Build history of the part. All positions in model axes, mm. A direction names the side the tool comes from. Round coordinates to 2 decimals unless told otherwise and drop trailing zeros. Write each loop counter-clockwise with the first axis right and the second up, starting at its lowest first coordinate (ties: lowest second). Pieces come first, ordered by that corner, then holes.
1) Saw through at D-D (z = 3.7). Write the cut outline in (x, y), plus the area to 3 significant figures.
2) Which spindle directions (+Z, -Z, +X, -X, +Y, -Y) get a long thin tool onto all of the face, cutting with end or side? Do faces 4 (the flat face through (12.3, -12.3, 3)), 5 (the cylindrical face through (-12.5, 11.07, 1.52)). Say none if no direction does.
3) Saw through at B-B (x = 0). Write the cut outline in (y, z), plus the area to 3 significant figures.
4) Flat gauge pins, fed straight in: pin 1 (2.5 mm diameter, centred on x = -11, y = -11, fed in from -Z); pin 2 (1.8 mm diameter, centred on x = 9.5, y = 10, fed in from +Z); pin 3 (8 mm diameter, centred on x = -11, y = 11, fed in from +Z). Where does each tip first touch, or does it go through?
5) Pull direction Y, two halves, no side cores. Call faces 1 (the flat face through (0, -15, 3)), 2 (the flat face through (-9.7, 9.7, 3)), 3 (the flat face through (0, 15, 3)): +Y half, -Y half, draft (parallel to the pull), parting line (faces both ways), or undercut.
6) Saw through at A-A (y = -11). Write the cut outline in (x, z).
7) Wall check: probe 1 along Y at (x, z) = (11, 5.25); probe 2 along Y at (x, z) = (-11, 1.45); probe 3 along X at (y, z) = (10.5, 1.65). Give the ranges that are in metal, low to high.
from build123d import *

# Parameters (mm, degrees)
SKETCH1_W           = 30
SKETCH1_H           = 30
SKETCH1_R           = 9.5
BOSS_EXTRUDE1_DEPTH = 6
SKETCH3_R           = 1.5
CUT_EXTRUDE2_DEPTH  = 7
SKETCH4_R           = 3
CUT_EXTRUDE3_DEPTH  = 3
FILLET1_R           = 3


with BuildPart() as part:
    # Sketch1 → Boss-Extrude1 (new body)
    with BuildSketch(Plane.XY):
        Rectangle(SKETCH1_W, SKETCH1_H)
        Circle(SKETCH1_R, mode=Mode.SUBTRACT)
    extrude(amount=BOSS_EXTRUDE1_DEPTH)

    # Sketch3 → Cut-Extrude2 (cut, through all)
    with BuildSketch(Plane.XY.offset(6)):
        with Locations((-11, 11)):
            Circle(SKETCH3_R)
        with Locations((11, 11)):
            Circle(SKETCH3_R)
        with Locations((11, -11)):
            Circle(SKETCH3_R)
        with Locations((-11, -11)):
            Circle(SKETCH3_R)
    extrude(amount=-CUT_EXTRUDE2_DEPTH, mode=Mode.SUBTRACT)

    # Sketch4 → Cut-Extrude3 (cut)
    with BuildSketch(Plane.XY.offset(6)):
        with Locations((-11, 11)):
            Circle(SKETCH4_R)
        with Locations((11, 11)):
            Circle(SKETCH4_R)
        with Locations((11, -11)):
            Circle(SKETCH4_R)
        with Locations((-11, -11)):
            Circle(SKETCH4_R)
    extrude(amount=-CUT_EXTRUDE3_DEPTH, mode=Mode.SUBTRACT)

    # Fillet1
    fillet1_edges = [part.edges().sort_by_distance(p)[0] for p in [
        (15, -15, 3),
        (-15, -15, 3),
        (-15, 15, 3),
        (15, 15, 3),
    ]]
    fillet(fillet1_edges, radius=FILLET1_R)


solid = part.part
Evaluation:
1. outline: (-15, -12) arc R3 ccw to (-12, -15) - (12, -15) arc R3 ccw to (15, -12) - (15, 12) arc R3 ccw to (12, 15) - (-12, 15) arc R3 ccw to (-15, 12) - close; hole circle Ø6 at (-11, -11); hole circle Ø6 at (-11, 11); hole circle Ø19 at (0, 0); hole circle Ø6 at (11, -11); hole circle Ø6 at (11, 11)
1. area: 496 mm2
2. face 4: +Z
2. face 5: +Z, -Z
3. outline: (-15, 0) - (-9.5, 0) - (-9.5, 6) - (-15, 6) - close; (9.5, 0) - (15, 0) - (15, 6) - (9.5, 6) - close
3. area: 66.0 mm2
4. pin 1: passes through
4. pin 2: stops at z = 3
4. pin 3: stops at z = 6
5. face 1: -Y half
5. face 2: undercut
5. face 3: +Y half
6. outline: (-15, 0) - (-12.5, 0) - (-12.5, 3) - (-14, 3) - (-14, 6) - (-15, 6) - close; (-9.5, 0) - (9.5, 0) - (9.5, 3) - (8, 3) - (8, 6) - (-8, 6) - (-8, 3) - (-9.5, 3) - close; (12.5, 0) - (15, 0) - (15, 6) - (14, 6) - (14, 3) - (12.5, 3) - close
7. probe 1: y = -15 to -14, -8 to 8, 14 to 15
7. probe 2: y = -15 to -12.5, -9.5 to 9.5, 12.5 to 15
7. probe 3: x = -15 to -12.41, -9.59 to 9.59, 12.41 to 15
